Read the model definition and answer for the solid it produces. Units are mm, in the model's axes. Face numbers are marked on the shaded views. A direction names the side the tool comes from. Round coordinates to 2 decimals unless told otherwise and drop trailing zeros. Loops run counter-clockwise (first coordinate to the right, second up) from the corner with the lowest first, then second, coordinate; pieces in that order, holes last. Notation, with made-up numbers: M 64,-37.5 L 113,-37.5 A16 ccw 113,-10.5 Z; hole C 24,-22 d10. An arc over 180 degrees is marked long. Answer as CSV lines item,"result".
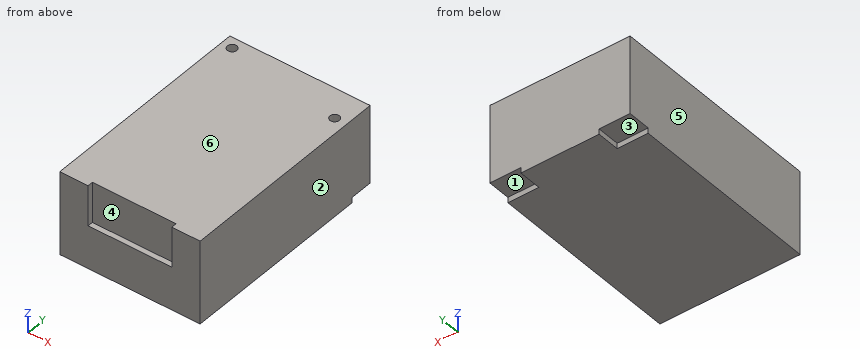
```python
from build123d import *

# Parameters (mm, degrees)
ESQUISSE1_W             = 52
ESQUISSE1_H             = 80
ESQUISSE1_R             = 1.75
BOSS_EXTRU_1_DEPTH      = 31
ESQUISSE3_W             = 31
ESQUISSE3_H             = 15
ENL_V_MAT_EXTRU_3_DEPTH = 2
ESQUISSE1_2_R           = 1.75
BOSS_EXTRU_3_DEPTH      = 25
ESQUISSE2_W             = 11.5
ESQUISSE2_H             = 8.5
ENL_V_MAT_EXTRU_1_DEPTH = 2


with BuildPart() as part:
    # Esquisse1 → Boss.-Extru.1 (new body)
    with BuildSketch(Plane.XY):
        Rectangle(ESQUISSE1_W, ESQUISSE1_H)
        with Locations((21.5, 29)):
            Circle(ESQUISSE1_R, mode=Mode.SUBTRACT)
        with Locations((-22, 36)):
            Circle(ESQUISSE1_R, mode=Mode.SUBTRACT)
    extrude(amount=BOSS_EXTRU_1_DEPTH)

    # Esquisse3 → Enlèv. mat.-Extru.3 (cut)
    with BuildSketch(Plane.XZ.offset(40)):
        with Locations((0, 23.5)):
            Rectangle(ESQUISSE3_W, ESQUISSE3_H)
    extrude(amount=-ENL_V_MAT_EXTRU_3_DEPTH, mode=Mode.SUBTRACT)

    # Esquisse1<2> → Boss.-Extru.3 (add)
    with BuildSketch(Plane.XY):
        with Locations((21.5, 29)):
            Circle(ESQUISSE1_2_R)
        with Locations((-22, 36)):
            Circle(ESQUISSE1_2_R)
    extrude(amount=BOSS_EXTRU_3_DEPTH)

    # Esquisse2 → Enlèv. mat.-Extru.1 (cut)
    with BuildSketch(Plane(origin=(0, 0, 0), x_dir=(-1, 0, 0), z_dir=(0, 0, -1))):
        with Locations((-20.25, 35.75)):
            Rectangle(ESQUISSE2_W, ESQUISSE2_H)
        with Locations((20.25, 35.75)):
            Rectangle(ESQUISSE2_W, ESQUISSE2_H)
    extrude(amount=-ENL_V_MAT_EXTRU_1_DEPTH, mode=Mode.SUBTRACT)


solid = part.part
```
1) Each of these flat-tipped pins is pushed along its axis until it touches: P1, Ø3, axis at x = -21.5, y = 36, coming from the +Z side; P2, Ø2.5, axis at x = -19.5, y = 35.5, coming from the -Z side; P3, Ø4, axis at x = -8, z = 25, coming from the -Y side; P4, Ø1.6, axis at y = 34, z = 0.5, coming from the -X side. Where does it stop, or does it pass through?
Evaluation:
P1,"stops at z = 31"
P2,"stops at z = 2"
P3,"stops at y = -38"
P4,"stops at x = -14.5"
2) A tool of negligible diameter and unlimited length cuts with its end or side. For the marked faces 1, 2 and 3, from which of +Z, -Z, +X, -X, +Y, -Y can it reach the whole face along a straight path? Write none if from no direction.
Evaluation:
face 1,"-Z, +X, +Y"
face 2,"+Z, -Z, +X, +Y, -Y"
face 3,"-Z, -X, +Y"
3) Find section A-A, the plane y = 36. Give the vertices of the cut face in (x, z).
Evaluation:
outline,"M -26,2 L -14.5,2 L -14.5,0 L 14.5,0 L 14.5,2 L 26,2 L 26,31 L -20.25,31 L -20.25,25 L -23.75,25 L -23.75,31 L -26,31 Z"
4) Determine the mould class of the marked faces 4, 5 and 6 for opening direction X: released by +X, released by -X, zero draft, split by the parting line, or undercut.
Evaluation:
face 4,"undercut"
face 5,"released by -X"
face 6,"zero draft"
5) Straight lines are drawn through the part: line 1 (Y direction, x = 21.5, z = 27.85); line 2 (Y direction, x = -22, z = 27.35); line 3 (Z direction, x = -19.5, y = 33.5). For each, find the intervals that lie inside material, in ascending order.
Evaluation:
line 1,"y = -40 to 27.25, 30.75 to 40"
line 2,"y = -40 to 34.25, 37.75 to 40"
line 3,"z = 2 to 31"
6) Find section B-B, the plane x = 21.5. Give the vertices of the cut face in (y, z).
Evaluation:
outline,"M -40,0 L 31.5,0 L 31.5,2 L 40,2 L 40,31 L 30.75,31 L 30.75,25 L 27.25,25 L 27.25,31 L -40,31 Z"
